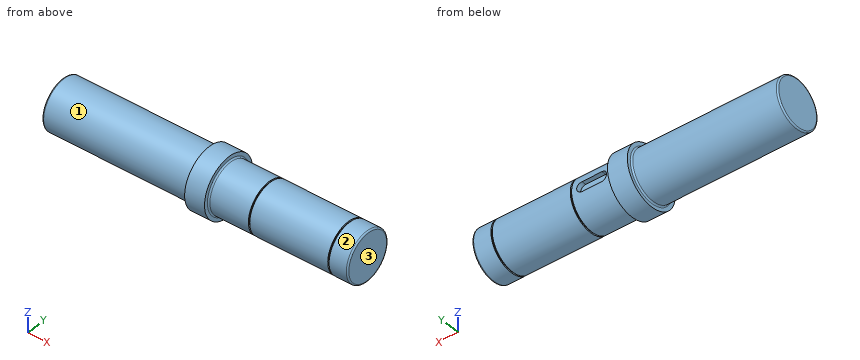
from build123d import *

# Parameters (mm, degrees)
CUT_EXTRUDE1_START = 25.4
CUT_EXTRUDE1_DEPTH = 185.822406037


with BuildPart() as part:
    # Sketch1 one side → Revolve1 (revolve)
    with BuildSketch(Plane(origin=(0, 0, 0), x_dir=(1, 0, 0), z_dir=(0, 1, 0)), mode=Mode.PRIVATE) as revolve1_sk:
        with BuildLine():
            Line((-186.944, 29.972), (-186.944, 0))
            Line((-186.944, 0), (0, 0))
            Line((0, 0), (31.75, 0))
            Line((31.75, 0), (69.85, 0))
            Line((69.85, 0), (203.2, 0))
            Line((203.2, 0), (203.2, 29.972))
            ThreePointArc((203.2, 29.972), (202.679235857, 31.229235857), (201.422, 31.75))
            Line((201.422, 31.75), (179.4002, 31.75))
            Line((179.4002, 31.75), (179.4002, 30.0228))
            Line((179.4002, 30.0228), (177.673, 30.0228))
            Line((177.673, 30.0228), (177.673, 31.75))
            Line((177.673, 31.75), (78.0542, 31.75))
            Line((78.0542, 31.75), (78.0542, 30.0228))
            Line((78.0542, 30.0228), (76.327, 30.0228))
            Line((76.327, 30.0228), (76.327, 31.75))
            Line((76.327, 31.75), (27.178, 31.75))
            ThreePointArc((27.178, 31.75), (25.920764143, 32.270764143), (25.4, 33.528))
            Line((25.4, 33.528), (25.4, 38.1))
            Line((25.4, 38.1), (0, 38.1))
            Line((0, 38.1), (0, 33.528))
            ThreePointArc((0, 33.528), (-0.520764143, 32.270764143), (-1.778, 31.75))
            Line((-1.778, 31.75), (-185.166, 31.75))
            ThreePointArc((-185.166, 31.75), (-186.423235857, 31.229235857), (-186.944, 29.972))
        make_face()
    revolve(revolve1_sk.sketch.rotate(Axis((0, 0, 0), (1, 0, 0)), 180), axis=Axis((0, 0, 0), (1, 0, 0)))

    # Sketch1_4 → Cut-Extrude1 (cut, through all)
    with BuildSketch(Plane(origin=(0, 0, 0), x_dir=(1, 0, 0), z_dir=(0, 1, 0)).offset(CUT_EXTRUDE1_START)):
        with BuildLine():
            Line((38.1, 6.35), (63.5, 6.35))
            ThreePointArc((63.5, 6.35), (69.85, 0), (63.5, -6.35))
            Line((63.5, -6.35), (38.1, -6.35))
            ThreePointArc((38.1, -6.35), (31.75, 0), (38.1, 6.35))
        make_face()
    extrude(amount=CUT_EXTRUDE1_DEPTH, mode=Mode.SUBTRACT)


solid = part.part
Here's how the part is built. I have some questions about the finished solid (model axes, mm). Face numbers are marked on the shaded views. A direction names the side the tool comes from. Give positions to 0.01 mm unless a question says otherwise; leave off trailing zeros. Order: outer loops, then holes, each group sorted by start corner. A loop starts at its lowest first (then second) coordinate and runs counter-clockwise, first axis right, second up. Notation, with made-up numbers: (25.5, 12) -> (76.5, 12) arc R28 ccw to (76.5, 48) -> close; hole circle Ø4 at (49.25, 33). An arc over 180 degrees is marked (long way). Use a Markdown table: item, result. Add a question column.
Item 1: Will these pins go through, and if not, where does the flat tip stop? pin 1 (1.5 mm diameter, centred on x = 24.5, y = -27, fed in from -Z); pin 2 (2 mm diameter, centred on x = 13.5, z = -5.5, fed in from -Y); pin 3 (8 mm diameter, centred on x = 100.5, z = 4.5, fed in from +Y).
Item 2: I need wall thicknesses on line 1 (X direction, y = -27.5, z = -12.5); line 2 (X direction, y = -35, z = 3); line 3 (Z direction, x = -102, y = -1). Which ranges of each line are inside material? Lowest first, please.
Item 3: For the marked faces 1, 2 and 3, which set-ups out of +Z, -Z, +X, -X, +Y, -Y let a thin tool reach every point of the face, with its end or its side?
Item 4: Imagine slicing it at B-B on x = 46. Please give me the cut outline in (y, z).
Item 5: Imagine slicing it at A-A on x = 139. Please give me the cut outline in (y, z).
Data:
| question | item | result |
|---|---|---|
| 1 | pin 1 | stops at z = -27.61 |
| 1 | pin 2 | stops at y = -37.83 |
| 1 | pin 3 | stops at y = 31.75 |
| 2 | line 1 | x = -186.93 to 76.33, 78.05 to 177.67, 179.4 to 203.18 |
| 2 | line 2 | x = 0 to 25.4 |
| 2 | line 3 | z = -31.73 to 31.73 |
| 3 | face 1 | -X |
| 3 | face 2 | +X |
| 3 | face 3 | +Z, -Z, +X, +Y, -Y |
| 4 | outline | (25.4, -6.35) -> (25.4, 6.35) -> (31.11, 6.35) arc R31.75 ccw (long way) to (31.11, -6.35) -> close |
| 5 | outline | circle Ø63.5 at (0, 0) |
